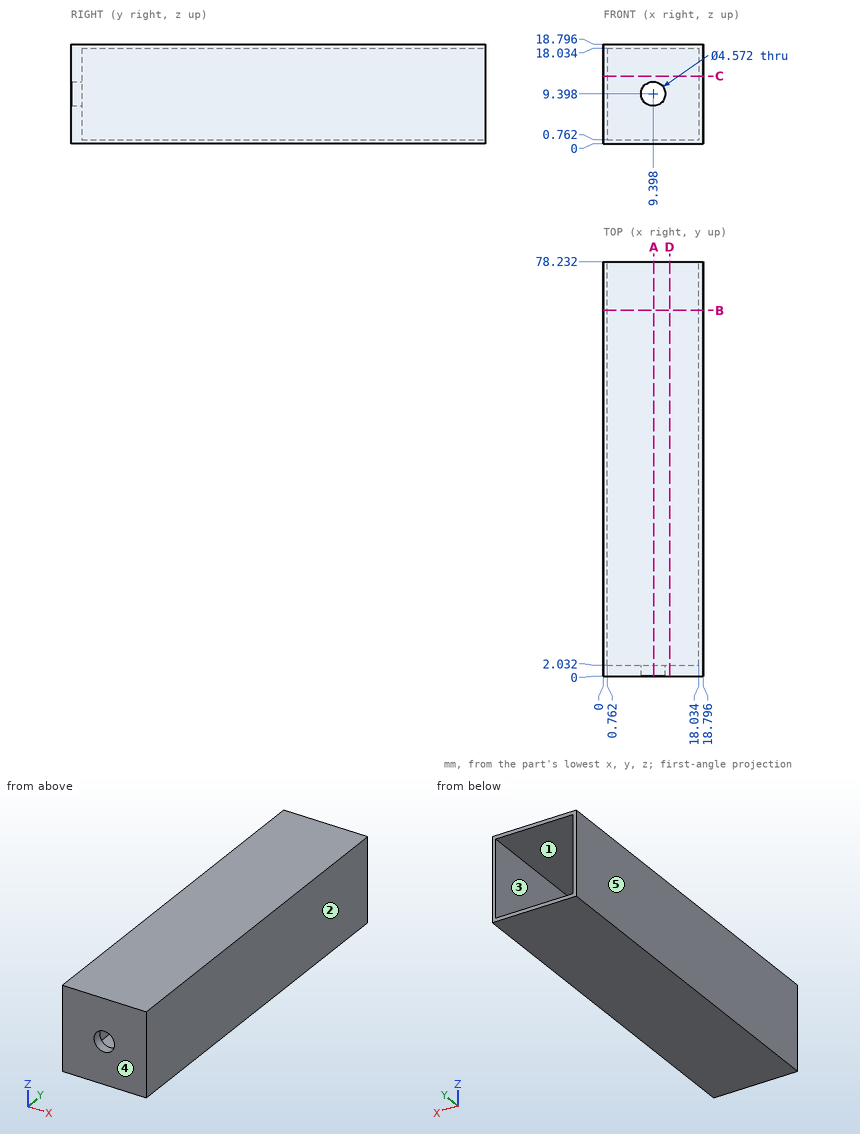
Could you check a few things on this drawing? It's one solid part, dimensions in mm from its lowest x, y, z. A direction names the side the tool comes from. Give positions to 0.01 mm unless a question says otherwise; leave off trailing zeros. Order: outer loops, then holes, each group sorted by start corner. A loop starts at its lowest first (then second) coordinate and runs counter-clockwise, first axis right, second up.
1. Suppose I cut it at D-D (x = 12.5). Write out the boundary of the cut face in (y, z).
Answers below:
outline: (0, 0) - (78.23, 0) - (78.23, 0.76) - (2.03, 0.76) - (2.03, 18.03) - (78.23, 18.03) - (78.23, 18.8) - (0, 18.8) - close
2. Suppose I cut it at C-C (z = 12.75). Write out the boundary of the cut face in (x, y).
Answers below:
outline: (0, 0) - (18.8, 0) - (18.8, 78.23) - (18.03, 78.23) - (18.03, 2.03) - (0.76, 2.03) - (0.76, 78.23) - (0, 78.23) - close
3. Suppose I cut it at B-B (y = 69). Write out the boundary of the cut face in (x, z).
Answers below:
outline: (0, 0) - (18.8, 0) - (18.8, 18.8) - (0, 18.8) - close; hole (0.76, 0.76) - (18.03, 0.76) - (18.03, 18.03) - (0.76, 18.03) - close
4. Which directions (+Z, -Z, +X, -X, +Y, -Y) give clear straight access to the entire face, cutting with the end or side of a thin tool? Please do the marked faces 1 and 2.
Answers below:
face 1: +Y
face 2: +Z, -Z, +X, +Y, -Y
5. I need wall thicknesses on L1, parallel to Z at x = 5.25, y = 13.5; L2, parallel to Y at x = 15, z = 6.25. Which ranges of each line are inside material? Lowest first, please.
Answers below:
L1: z = 0 to 0.76, 18.03 to 18.8
L2: y = 0 to 2.03
6. Thinking about a two-plate mould opening in X: for the marked faces 3, 4 and 5, which applies, +X half, -X half, draft (parallel to the pull), parting line (faces both ways), or undercut?
Answers below:
face 3: undercut
face 4: draft
face 5: -X half
7. For pin 1 (6 mm diameter, centred on x = 10.5, z = 8, fed in from +Y), with a flat end and sliding along its axis, tell me the tip position at first contact or that it passes through.
Answers below:
pin 1: stops at y = 2.03
8. Suppose I cut it at A-A (x = 9.5). Write out the boundary of the cut face in (y, z), plus the area to 3 significant figures.
Answers below:
outline: (0, 0) - (78.23, 0) - (78.23, 0.76) - (2.03, 0.76) - (2.03, 7.11) - (0, 7.11) - close; (0, 11.68) - (2.03, 11.68) - (2.03, 18.03) - (78.23, 18.03) - (78.23, 18.8) - (0, 18.8) - close
area: 145 mm2
